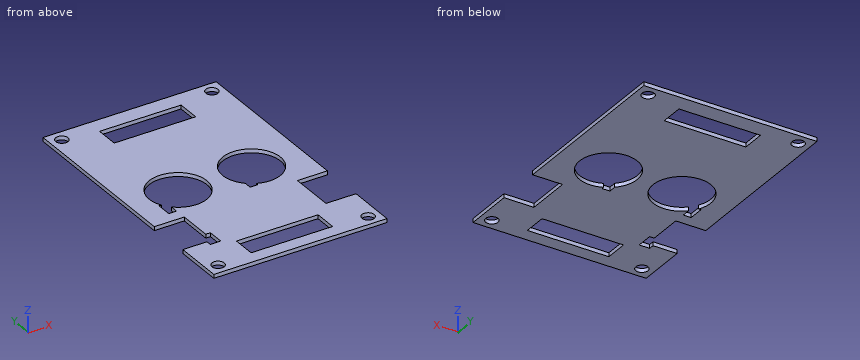
```python
from build123d import *

# Parameters (mm, degrees)
SKETCH1_R           = 1.6
BOSS_EXTRUDE1_DEPTH = 1
SKETCH5_W           = 2.05
SKETCH5_H           = 4
CUT_EXTRUDE1_DEPTH  = 4
SKETCH4_W           = 21.2
SKETCH4_H           = 6
CUT_EXTRUDE2_DEPTH  = 4
SKETCH2_R           = 7.5
CUT_EXTRUDE3_DEPTH  = 4


with BuildPart() as part:
    # Sketch1 → Boss-Extrude1 (new body)
    with BuildSketch(Plane.XY):
        Polygon((20.734205703, -15.283501687), (20.734205703, -27.983501687), (-24.265794297, -27.983501687), (-24.265794297, -15.283501687), (-17.985794297, -15.283501687), (-17.985794297, -16.633501687), (-15.265794297, -16.633501687), (-15.265794297, -12.383501687), (-16.465794297, -12.383501687), (-16.465794297, -3.583501687), (-24.265794297, -3.583501687), (-24.265794297, 42.016498313), (20.734205703, 42.016498313), (20.734205703, -3.583501687), (12.934205703, -3.583501687), (12.934205703, -15.283501687), align=None)
        with Locations((-21.265794297, 39.016498313)):
            Circle(SKETCH1_R, mode=Mode.SUBTRACT)
        with Locations((17.734205703, 39.016498313)):
            Circle(SKETCH1_R, mode=Mode.SUBTRACT)
        with Locations((-21.265794297, -24.983501687)):
            Circle(SKETCH1_R, mode=Mode.SUBTRACT)
        with Locations((17.734205703, -24.983501687)):
            Circle(SKETCH1_R, mode=Mode.SUBTRACT)
    extrude(amount=BOSS_EXTRUDE1_DEPTH)

    # Sketch5 → Cut-Extrude1 (cut)
    with BuildSketch(Plane.XY.offset(1)):
        with Locations((-17.540794297, 1.466498313)):
            Rectangle(SKETCH5_W, SKETCH5_H)
        with Locations((3.659205703, 1.566498313)):
            Rectangle(SKETCH5_W, SKETCH5_H)
    extrude(amount=-CUT_EXTRUDE1_DEPTH, mode=Mode.SUBTRACT)

    # Sketch4 → Cut-Extrude2 (cut)
    with BuildSketch(Plane.XY.offset(1)):
        with Locations((-1.765794297, -21.483501687)):
            Rectangle(SKETCH4_W, SKETCH4_H)
        with Locations((-1.765794297, 34.616498313)):
            Rectangle(SKETCH4_W, SKETCH4_H)
    extrude(amount=-CUT_EXTRUDE2_DEPTH, mode=Mode.SUBTRACT)

    # Sketch2 → Cut-Extrude3 (cut)
    with BuildSketch(Plane.XY.offset(1)):
        with Locations((-11.365794297, 7.016498313)):
            Circle(SKETCH2_R)
        with Locations((7.734205703, 7.016498313)):
            Circle(SKETCH2_R)
    extrude(amount=-CUT_EXTRUDE3_DEPTH, mode=Mode.SUBTRACT)


solid = part.part
```
Work out the finished part from the listing and answer in its coordinate system (mm). Round coordinates to 2 decimals unless told otherwise and drop trailing zeros. Order: outer loops, then holes, each group sorted by start corner. A loop starts at its lowest first (then second) coordinate and runs counter-clockwise, first axis right, second up.
Q1. A cutting plane is placed at B-B, the plane x = 10. Determine the outline of the cut face in (y, z).
Solution:
outline: (-27.98, 0) - (-0.13, 0) - (-0.13, 1) - (-27.98, 1) - close; (14.17, 0) - (42.02, 0) - (42.02, 1) - (14.17, 1) - close
Q2. A cutting plane is placed at D-D, the plane z = 0.15. Count the separate pieces of the cut face and the enclosed holes in it, then the cut area to 3 significant figures.
Solution:
separate pieces: 1
enclosed holes: 8
area: 2,310 mm2
Q3. Given pin 1 Ø4 at (x, y) = (-12.5, -16) entering from -Z; pin 2 Ø3 at (x, y) = (-21.27, 39.02) entering from -Z, each flat-ended and moving along its own axis, determine where each tip first touches the part or whether it passes through.
Solution:
pin 1: stops at z = 0
pin 2: passes through
Q4. Find the intervals of material crossed by line 1 along X through (y, z) = (7.5, 0.55); line 2 along Y through (x, z) = (-3, 0.3); line 3 along Y through (x, z) = (8, 0.7), in increasing order.
Solution:
line 1: x = -24.27 to -18.85, -3.88 to 0.25, 15.22 to 20.73
line 2: y = -27.98 to -24.48, -18.48 to 31.62, 37.62 to 42.02
line 3: y = -27.98 to -24.48, -18.48 to -0.48, 14.51 to 31.62, 37.62 to 42.02
Q5. A cutting plane is placed at C-C, the plane y = 2.5. Determine the outline of the cut face in (x, z), then the cut area to 3 significant figures.
Solution:
outline: (-24.27, 0) - (-18.57, 0) - (-18.57, 1) - (-24.27, 1) - close; (-5.38, 0) - (1.75, 0) - (1.75, 1) - (-5.38, 1) - close; (13.72, 0) - (20.73, 0) - (20.73, 1) - (13.72, 1) - close
area: 19.8 mm2
Q6. A cutting plane is placed at A-A, the plane x = 1.5. Determine the outline of the cut face in (y, z).
Solution:
outline: (-27.98, 0) - (-24.48, 0) - (-24.48, 1) - (-27.98, 1) - close; (-18.48, 0) - (2.85, 0) - (2.85, 1) - (-18.48, 1) - close; (11.19, 0) - (31.62, 0) - (31.62, 1) - (11.19, 1) - close; (37.62, 0) - (42.02, 0) - (42.02, 1) - (37.62, 1) - close
